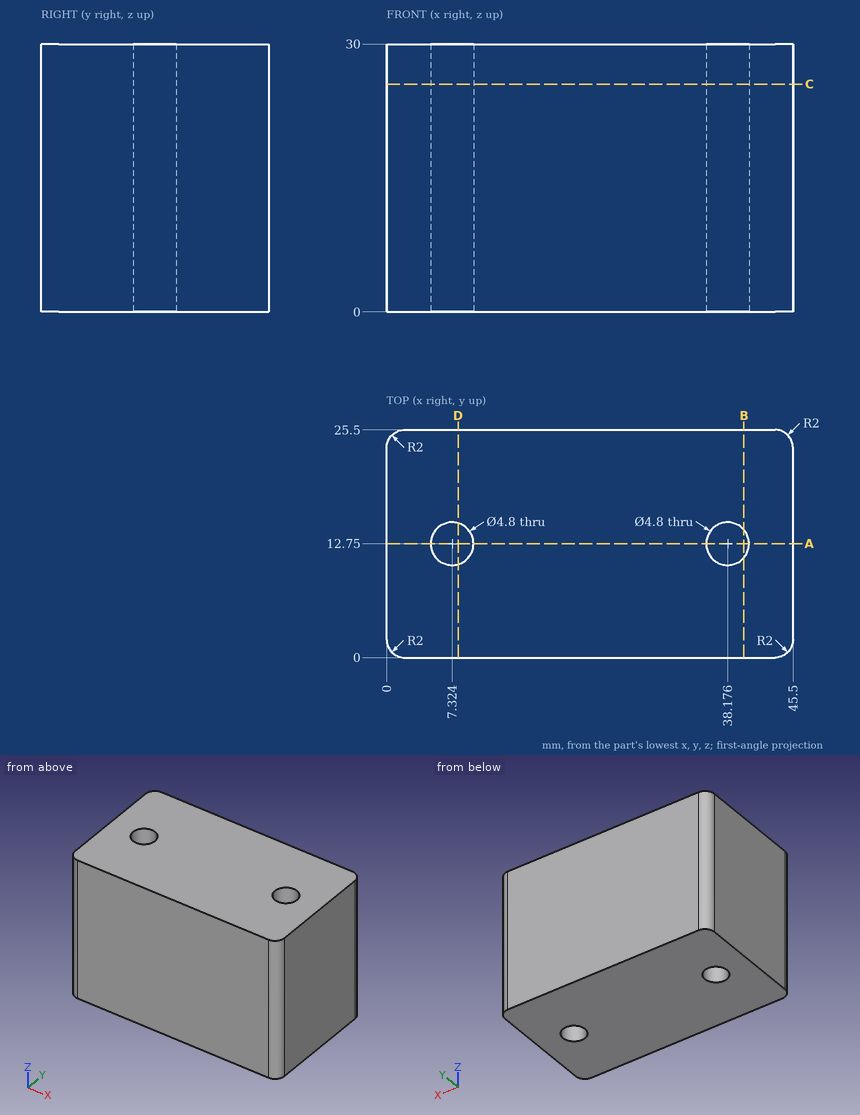
Geometry check sheet. Reference: drawing and pictorial views, mm from the part's lowest x, y, z. Give positions to 0.01 mm unless a question says otherwise; leave off trailing zeros. Order: outer loops, then holes, each group sorted by start corner. A loop starts at its lowest first (then second) coordinate and runs counter-clockwise, first axis right, second up. Notation, with made-up numbers: (61.25, 85) -> (95.25, 85) arc R17 cw to (95.25, 101) -> close; hole circle Ø5 at (30.5, -24.5). An arc over 180 degrees is marked (long way). Write each question's results on one line, items separated by ' | '. Start each with the question number.
(1) Sectioned sample at A-A (y = 12.75). Enter the section's corners in (x, z), plus the area to 3 significant figures.
(2) Gauge pin test, flat end, axial feed: P1, Ø2, axis at x = 5, y = 21, coming from the -Z side. Record the tip position at first contact, or that the pin passes through.
(3) Scan lines: line 1 (X direction, y = 11, z = 4) (1 decimal); line 2 (X direction, y = 12.25, z = 6.75); line 3 (Y direction, x = 8.5, z = 19.25). Record each from-to range of solid material in increasing order.
(4) Sectioned sample at D-D (x = 8). Enter the section's corners in (y, z), plus the area to 3 significant figures.
(5) Sectioned sample at B-B (x = 40). Enter the section's corners in (y, z).
(6) Sectioned sample at C-C (z = 25.5). Enter the section's corners in (x, y).
Answer below:
1) outline: (0, 0) -> (4.92, 0) -> (4.92, 30) -> (0, 30) -> close; (9.72, 0) -> (35.78, 0) -> (35.78, 30) -> (9.72, 30) -> close; (40.58, 0) -> (45.5, 0) -> (45.5, 30) -> (40.58, 30) -> close | area: 1,080 mm2
2) P1: z = 0
3) line 1: 0 to 5.7, 9 to 36.5, 39.8 to 45.5 | line 2: 0 to 4.98, 9.67 to 35.83, 40.52 to 45.5 | line 3: 0 to 10.66, 14.84 to 25.5
4) outline: (0, 0) -> (10.45, 0) -> (10.45, 30) -> (0, 30) -> close; (15.05, 0) -> (25.5, 0) -> (25.5, 30) -> (15.05, 30) -> close | area: 627 mm2
5) outline: (0, 0) -> (11.19, 0) -> (11.19, 30) -> (0, 30) -> close; (14.31, 0) -> (25.5, 0) -> (25.5, 30) -> (14.31, 30) -> close
6) outline: (0, 2) arc R2 ccw to (2, 0) -> (43.5, 0) arc R2 ccw to (45.5, 2) -> (45.5, 23.5) arc R2 ccw to (43.5, 25.5) -> (2, 25.5) arc R2 ccw to (0, 23.5) -> close; hole circle Ø4.8 at (7.32, 12.75); hole circle Ø4.8 at (38.18, 12.75)
